Design review of the part shown in the three views and the two pictorial views. Dimensions are in mm from the part's minimum x, y and z. A direction names the side the tool comes from. Coordinates: 2 decimals unless noted, no trailing zeros. Loops run counter-clockwise (first coordinate to the right, second up) from the corner with the lowest first, then second, coordinate; pieces in that order, holes last. Notation, with made-up numbers: (-14.75, 49) -> (-5.75, 49) arc R24 ccw to (-5.75, 84) -> close; hole circle Ø3 at (-25, 35.25). An arc over 180 degrees is marked (long way). One line per item, written item: value. Start each with the question number.
1. Add section C-C on x = 5. Write out the cut boundary in (y, z).
2. Insertion check: pin 1 (2 mm diameter, centred on x = 8, z = 19, fed in from +Y); pin 2 (0.6 mm diameter, centred on x = 1, y = 18, fed in from +Z); pin 3 (4.5 mm diameter, centred on x = 6.5, y = 16.5, fed in from +Z). Each pin has a flat end and moves straight along its axis. Give the tip position at first contact, or say it passes through.
3. Add section A-A on y = 15. Write out the cut boundary in (x, z), plus the area to 3 significant figures.
4. Draft analysis for pull direction X (two halves, no side actions). For the marked faces 1, 2 and 3, state which applies: pulls with the +X half, pulls with the -X half, needs draft (parallel to the pull), parting line crosses it, or undercut.
5. Machinability: for the marked faces 4, 5 and 6, which of the approach directions +Z, -Z, +X, -X, +Y, -Y give a long, thin tool a straight path to every point of the face, cutting with its end or side? Answer none if there is none.
6. Add section D-D on z = 18.5. Write out the cut boundary in (x, y).
7. For probe 1 along Y at (x, z) = (5, 3.1); probe 2 along X at (y, z) = (3, 15), list the stretches that pass through material, from the lowest coordinate up.
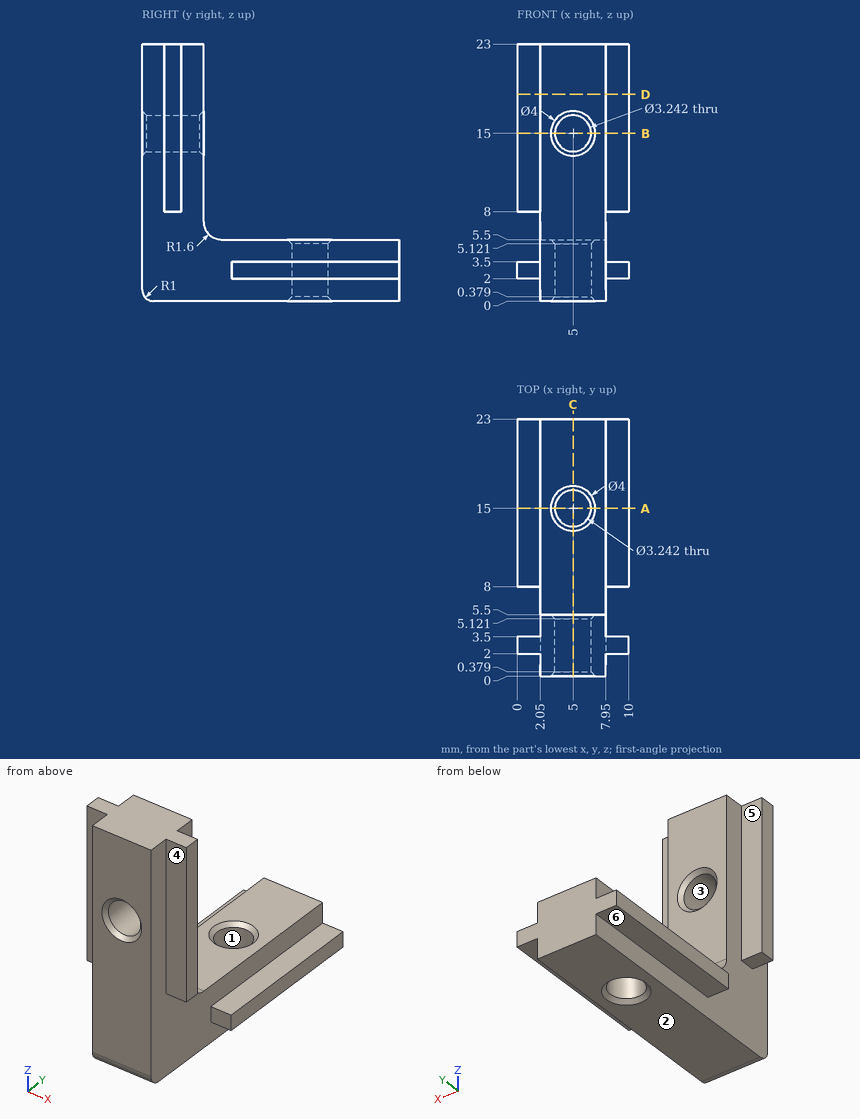
Worked answers:
1. outline: (0, 1) arc R1 ccw to (1, 0) -> (13, 0) -> (13.38, 0.38) -> (13.38, 5.12) -> (13, 5.5) -> (7.1, 5.5) arc R1.6 cw to (5.5, 7.1) -> (5.5, 13) -> (5.12, 13.38) -> (0.38, 13.38) -> (0, 13) -> close; (0, 17) -> (0.38, 16.62) -> (5.12, 16.62) -> (5.5, 17) -> (5.5, 23) -> (0, 23) -> close; (16.62, 0.38) -> (17, 0) -> (23, 0) -> (23, 5.5) -> (17, 5.5) -> (16.62, 5.12) -> close
2. pin 1: stops at y = 5.5
2. pin 2: stops at z = 3.5
2. pin 3: stops at z = 5.5
3. outline: (0, 2) -> (2.05, 2) -> (2.05, 0) -> (3, 0) -> (3.38, 0.38) -> (3.38, 5.12) -> (3, 5.5) -> (2.05, 5.5) -> (2.05, 3.5) -> (0, 3.5) -> close; (6.62, 0.38) -> (7, 0) -> (7.95, 0) -> (7.95, 2) -> (10, 2) -> (10, 3.5) -> (7.95, 3.5) -> (7.95, 5.5) -> (7, 5.5) -> (6.62, 5.12) -> close
3. area: 20.5 mm²
4. face 1: undercut
4. face 2: needs draft
4. face 3: undercut
5. face 4: +Z, -Z, +X, -Y
5. face 5: +Z, -Z, -X, +Y
5. face 6: -Z, -X, +Y, -Y
6. outline: (0, 2) -> (2.05, 2) -> (2.05, 0) -> (7.95, 0) -> (7.95, 2) -> (10, 2) -> (10, 3.5) -> (7.95, 3.5) -> (7.95, 5.5) -> (2.05, 5.5) -> (2.05, 3.5) -> (0, 3.5) -> close
7. probe 1: y = 0 to 13.38, 16.62 to 23
7. probe 2: x = 0 to 3.38, 6.62 to 10
